Geometry check sheet. Reference: the model listing, model coordinates, mm. A direction names the side the tool comes from. Round coordinates to 2 decimals unless told otherwise and drop trailing zeros. Write each loop counter-clockwise with the first axis right and the second up, starting at its lowest first coordinate (ties: lowest second). Pieces come first, ordered by that corner, then holes.
from build123d import *

# Parameters (mm, degrees)
F1_DEPTH        = 50
F2_W            = 25
F2_H            = 30
F3_DEPTH        = 50.001
F5_DEPTH        = 50
F6_W            = 42.5
F6_H            = 25
F7_DEPTH        = 50.001
F8_R            = 12.5
F9_DEPTH        = 5
F10_R           = 12.5
F11_DEPTH       = 5
F12_R           = 6
F13_DEPTH       = 201
F15_D           = 12
F17_DEPTH       = 5
F19_DEPTH       = 5
F21_D           = 10
F21_DEPTH       = 17.5
F21_CBORE_D     = 18
F21_CBORE_DEPTH = 2
F21_TIP         = 3.0043030951
F23_D           = 10
F23_DEPTH       = 17.5
F23_CBORE_D     = 18
F23_CBORE_DEPTH = 2
F23_TIP         = 3.0043030951


# Not quite as in the source:
# - an extrude ends at something that could not be found from the text; its depth is read off the source's solid


with BuildPart() as f1:
    # F0 (on Front) → F1 (new body)
    with BuildSketch(Plane.XZ):
        with BuildLine():
            Line((25, 25), (0, 25))
            ThreePointArc((0, 25), (-25, 0), (0, -25))
            Line((0, -25), (25, -25))
            Line((25, -25), (25, -17))
            Line((25, -17), (50, -17))
            Line((50, -17), (50, -25))
            Line((50, -25), (62, -25))
            Line((62, -25), (62, 0))
            Line((62, 0), (62, 25))
            Line((62, 25), (50, 25))
            Line((50, 25), (50, 17))
            Line((50, 17), (25, 17))
            Line((25, 17), (25, 25))
        make_face()
    extrude(amount=F1_DEPTH)

    # F2 (on face) → F3 (cut, through all)
    with BuildSketch(Plane.XY.offset(25)):
        with Locations((-12.5, -25)):
            Rectangle(F2_W, F2_H)
        with Locations((12.5, -25)):
            Rectangle(F2_W, F2_H)
        with Locations((37.5, -25)):
            Rectangle(F2_W, F2_H)
    extrude(amount=-F3_DEPTH, mode=Mode.SUBTRACT)

    # F4 (on face) → F5 (join)
    with BuildSketch(Plane.XY.offset(25)):
        with BuildLine():
            Line((62, -50), (96.5075043991, -36.6590052789))
            ThreePointArc((96.5075043991, -36.6590052789), (104.5, -25), (96.5075043991, -13.3409947211))
            Line((96.5075043991, -13.3409947211), (62, 0))
            Line((62, 0), (62, -50))
        make_face()
    extrude(amount=-F5_DEPTH)

    # F6 (on face) → F7 (cut, through all)
    with BuildSketch(Plane.XZ.offset(50)):
        with Locations((83.25, 0)):
            Rectangle(F6_W, F6_H)
    extrude(amount=-F7_DEPTH, mode=Mode.SUBTRACT)

    # F8 (on face) → F9 (join)
    with BuildSketch(Plane.XZ.offset(50)):
        Circle(F8_R)
    extrude(amount=F9_DEPTH)

    # F10 (on face) → F11 (join)
    with BuildSketch(Plane(origin=(0, 0, 0), x_dir=(-1, 0, 0), z_dir=(0, 1, 0))):
        Circle(F10_R)
    extrude(amount=F11_DEPTH)

    # F12 (on face) → F13 (cut, through all)
    with BuildSketch(Plane(origin=(0, 5, 0), x_dir=(-1, 0, 0), z_dir=(0, 1, 0))):
        Circle(F12_R)
    extrude(amount=F13_DEPTH, mode=Mode.SUBTRACT)

    # F15 (through all)
    with Locations(Plane.XZ.offset(55)):
        with Locations((0, 0)):
            Hole(F15_D / 2)

    # F16 (on face) → F17 (join)
    with BuildSketch(Plane.XY.offset(-12.5)):
        with BuildLine():
            ThreePointArc((96.5075043991, -36.6590052789), (102.3100389182, -32.0677505266), (104.5, -25))
            ThreePointArc((104.5, -25), (102.3100389182, -17.9322494734), (96.5075043991, -13.3409947211))
            ThreePointArc((96.5075043991, -13.3409947211), (79.5, -25), (96.5075043991, -36.6590052789))
        make_face()
    extrude(amount=F17_DEPTH)

    # F18 (on face) → F19 (join)
    with BuildSketch(Plane(origin=(0, 0, 12.5), x_dir=(1, 0, 0), z_dir=(0, 0, -1))):
        with BuildLine():
            ThreePointArc((96.5075043991, 13.3409947211), (102.3100389182, 17.9322494734), (104.5, 25))
            ThreePointArc((104.5, 25), (102.3100389182, 32.0677505266), (96.5075043991, 36.6590052789))
            ThreePointArc((96.5075043991, 36.6590052789), (79.5, 25), (96.5075043991, 13.3409947211))
        make_face()
    extrude(amount=F19_DEPTH)

    # F21
    with Locations(Plane.XY.offset(25)):
        with Locations((92, -25)):
            CounterBoreHole(F21_D / 2, F21_CBORE_D / 2, F21_CBORE_DEPTH, depth=F21_DEPTH)
            with Locations((0, 0, -(F21_DEPTH + F21_TIP / 2))):  # 118° drill point
                Cone(0, F21_D / 2, F21_TIP, mode=Mode.SUBTRACT)

    # F23
    with Locations(Plane(origin=(0, 0, -25), x_dir=(1, 0, 0), z_dir=(0, 0, -1))):
        with Locations((92, 25)):
            CounterBoreHole(F23_D / 2, F23_CBORE_D / 2, F23_CBORE_DEPTH, depth=F23_DEPTH)
            with Locations((0, 0, -(F23_DEPTH + F23_TIP / 2))):  # 118° drill point
                Cone(0, F23_D / 2, F23_TIP, mode=Mode.SUBTRACT)


solid = f1.part
1. Section check B-B (x = 23.5). Record the cut outline in (y, z).
2. Section check A-A (z = 0). Record the cut outline in (x, y), plus the area to 3 significant figures.
3. Depth check by flat-ended pin: pin 1 Ø3 at (x, y) = (34.5, -4) entering from -Z; pin 2 Ø11 at (x, y) = (33, -44) entering from +Z; pin 3 Ø3 at (x, y) = (91.5, -29.5) entering from +Z. Enter the tip coordinate at first touch or a pass-through.
4. Release check for a two-part mould opening along Y. For faces 5 (the face through (100.584, -27.703, -24.014)), 6 (the face through (18, 0, 0)), 7 (the face through (87.381, -23.085, -15.142)), 8 (the face through (38, -45, 17)) record: +Y half, -Y half, draft (parallel to the pull), parting line (faces both ways), or undercut.
5. Section check C-C (z = 21.5). Record the cut outline in (x, y).
6. Access from +Z, -Z, +X, -X, +Y, -Y to the whole of each face (thin tool, end or side, straight path). Record for faces 1 (the face through (96, -29, 23)), 2 (the face through (-11.923, 2.465, 3.755)), 3 (the face through (25, -5, -21)), 4 (the face through (25, -5, 21)).
7. Section check D-D (y = -2). Record the cut outline in (x, z), plus the area to 3 significant figures.
8. Scan lines: line 1 along Y through (x, z) = (18, 18.5); line 2 along X through (y, z) = (-25, -18); line 3 along Z through (x, y) = (0, 1.5). Record each from-to range of solid material in increasing order.
Results below:
1. outline: (-50, -25) - (-40, -25) - (-40, 25) - (-50, 25) - close; (-10, -25) - (0, -25) - (0, 25) - (-10, 25) - close
2. outline: (-25, -50) - (-12.5, -50) - (-12.5, -55) - (-6, -55) - (-6, -40) - (-25, -40) - close; (-25, -10) - (-6, -10) - (-6, 5) - (-12.5, 5) - (-12.5, 0) - (-25, 0) - close; (6, -55) - (12.5, -55) - (12.5, -50) - (62, -50) - (62, 0) - (12.5, 0) - (12.5, 5) - (6, 5) - (6, -10) - (50, -10) - (50, -40) - (6, -40) - close
2. area: 1,990 mm2
3. pin 1: stops at z = -17
3. pin 2: stops at z = 17
3. pin 3: stops at z = 23
4. face 5: undercut
4. face 6: +Y half
4. face 7: undercut
4. face 8: draft
5. outline: (-12.76, -50) - (25, -50) - (25, -40) - (-12.76, -40) - close; (-12.76, -10) - (25, -10) - (25, 0) - (-12.76, 0) - close; (50, -50) - (62, -50) - (96.51, -36.66) arc R12.5 ccw to (96.51, -13.34) - (62, 0) - (50, 0) - close; hole circle Ø10 at (92, -25)
6. face 1: +Z
6. face 2: +Y
6. face 3: -Z, +Y, -Y
6. face 4: +Z, +Y, -Y
7. outline: (0, -25) - (25, -25) - (25, -17) - (50, -17) - (50, -25) - (67.17, -25) - (67.17, -12.5) - (62, -12.5) - (62, 12.5) - (67.17, 12.5) - (67.17, 25) - (50, 25) - (50, 17) - (25, 17) - (25, 25) - (0, 25) arc R25 ccw to start; hole circle Ø12 at (0, 0)
7. area: 3,700 mm2
8. line 1: y = -50 to -40, -10 to 0
8. line 2: x = 50 to 87, 97 to 104.5
8. line 3: z = -12.5 to -6, 6 to 12.5
